```python
from build123d import *

# Parameters (mm, degrees)
SKETCH_W     = 60.2
SKETCH_H     = 8.2
PAD_DEPTH    = 0.7
SKETCH001_R  = 1
POCKET_DEPTH = 0.701
SKETCH002_W  = 8.2
SKETCH002_H  = 8.2
PAD001_DEPTH = 3
SKETCH003_R  = 3.25
PAD002_DEPTH = 5.6
SKETCH004_R  = 5
PAD003_DEPTH = 2.4
SKETCH005_R  = 4.5
PAD004_DEPTH = 0.6
SKETCH006_W  = 6.08
SKETCH006_H  = 7.5
PAD005_DEPTH = 3.2


with BuildPart() as part:
    # Sketch → Pad (new body)
    with BuildSketch(Plane.XY):
        Rectangle(SKETCH_W, SKETCH_H)
    extrude(amount=PAD_DEPTH)

    # Sketch001 → Pocket (cut, through all)
    with BuildSketch(Plane.XY.offset(0.7)):
        with Locations((-28.1, 2.1)):
            Circle(SKETCH001_R)
        with Locations((-28.1, -2.1)):
            Circle(SKETCH001_R)
        with Locations((22.4, 2.1)):
            Circle(SKETCH001_R)
    extrude(amount=-POCKET_DEPTH, mode=Mode.SUBTRACT)

    # Sketch002 → Pad001 (new body)
    with BuildSketch(Plane.XY.offset(0.7)):
        with Locations((2.4, 0)):
            Rectangle(SKETCH002_W, SKETCH002_H)
    extrude(amount=PAD001_DEPTH)

    # Sketch003 → Pad002 (new body)
    with BuildSketch(Plane.XY.offset(3.7)):
        with Locations((2.4, 0)):
            Circle(SKETCH003_R)
    extrude(amount=PAD002_DEPTH)

    # Sketch004 → Pad003 (new body)
    with BuildSketch(Plane.XY.offset(9.3)):
        with Locations((2.4, 0)):
            Circle(SKETCH004_R)
    extrude(amount=PAD003_DEPTH)

    # Sketch005 → Pad004 (new body)
    with BuildSketch(Plane.XY.offset(11.7)):
        with Locations((2.4, 0)):
            Circle(SKETCH005_R)
    extrude(amount=PAD004_DEPTH)

    # Sketch006 → Pad005 (new body)
    with BuildSketch(Plane.XY.offset(0.7)):
        with Locations((29.64, 0)):
            Rectangle(SKETCH006_W, SKETCH006_H)
    extrude(amount=PAD005_DEPTH)


solid = part.part
```
Can you work these out from the model? Positions are in its coordinate system, mm. A direction names the side the tool comes from. Coordinates: 2 decimals unless noted, no trailing zeros. Loops run counter-clockwise (first coordinate to the right, second up) from the corner with the lowest first, then second, coordinate; pieces in that order, holes last.
1) Imagine slicing it at B-B on z = 1.25. List the corners of the cut face in (x, y) for me.
2) For pin 1 (2.5 mm diameter, centred on x = 21, y = -0.5, fed in from +Z); pin 2 (1.8 mm diameter, centred on x = -11.5, z = 2.5, fed in from -Y); pin 3 (3 mm diameter, centred on x = -4, z = 1, fed in from +Y); pin 4 (2.5 mm diameter, centred on y = 1.5, z = 2.5, fed in from -X), each with a flat end and sliding along its axis, tell me the tip position at first contact or that it passes through.
3) Imagine slicing it at C-C on y = -2.1. List the corners of the cut face in (x, z) for me, plus the area to 3 significant figures.
4) Which directions (+Z, -Z, +X, -X, +Y, -Y) give clear straight access to the entire face, cutting with the end or side of a thin tool? Please do faces 1 (the flat face through (6.5, 0, 2)), 2 (the flat face through (30, 3.75, 2)), 3 (the flat face through (4, 3, 3.7)).
5) Thinking about a two-plate mould opening in Z: for faces 4 (the cylindrical face through (-27.146, 2.4, 0.355)), 5 (the cylindrical face through (5.5, 0.98, 6.46)), 6 (the flat face through (2, 0, 12.3)), which applies, pulls with the +Z half, pulls with the -Z half, needs draft (parallel to the pull), parting line crosses it, or undercut?
6) Imagine slicing it at D-D on x = 2.4. List the corners of the cut face in (y, z) for me, plus the area to 3 significant figures.
7) Imagine slicing it at A-A on x = 22.4. List the corners of the cut face in (y, z) for me, plus the area to 3 significant figures.
8) I need wall thicknesses on probe 1 along Y at (x, z) = (-28.1, 0.55); probe 2 along Y at (x, z) = (22.4, 0.5); probe 3 along Z at (x, y) = (-28, 3.75). Which ranges of each line are inside material? Lowest first, please.
Completed:
1. outline: (-1.7, -4.1) - (6.5, -4.1) - (6.5, 4.1) - (-1.7, 4.1) - close; (26.6, -3.75) - (32.68, -3.75) - (32.68, 3.75) - (26.6, 3.75) - close
2. pin 1: stops at z = 0.7
2. pin 2: passes through
2. pin 3: stops at y = 4.1
2. pin 4: stops at x = -1.7
3. outline: (-30.1, 0) - (-29.1, 0) - (-29.1, 0.7) - (-30.1, 0.7) - close; (-27.1, 0) - (30.1, 0) - (30.1, 0.7) - (32.68, 0.7) - (32.68, 3.9) - (26.6, 3.9) - (26.6, 0.7) - (6.5, 0.7) - (6.5, 3.7) - (4.88, 3.7) - (4.88, 9.3) - (6.94, 9.3) - (6.94, 11.7) - (6.38, 11.7) - (6.38, 12.3) - (-1.58, 12.3) - (-1.58, 11.7) - (-2.14, 11.7) - (-2.14, 9.3) - (-0.08, 9.3) - (-0.08, 3.7) - (-1.7, 3.7) - (-1.7, 0.7) - (-27.1, 0.7) - close
3. area: 139 mm2
4. face 1: +Y, -Y
4. face 2: +Z, +X, +Y
4. face 3: none
5. face 4: needs draft
5. face 5: undercut
5. face 6: pulls with the +Z half
6. outline: (-5, 9.3) - (-3.25, 9.3) - (-3.25, 3.7) - (-4.1, 3.7) - (-4.1, 0) - (4.1, 0) - (4.1, 3.7) - (3.25, 3.7) - (3.25, 9.3) - (5, 9.3) - (5, 11.7) - (4.5, 11.7) - (4.5, 12.3) - (-4.5, 12.3) - (-4.5, 11.7) - (-5, 11.7) - close
6. area: 96.1 mm2
7. outline: (-4.1, 0) - (1.1, 0) - (1.1, 0.7) - (-4.1, 0.7) - close; (3.1, 0) - (4.1, 0) - (4.1, 0.7) - (3.1, 0.7) - close
7. area: 4.34 mm2
8. probe 1: y = -4.1 to -3.1, -1.1 to 1.1, 3.1 to 4.1
8. probe 2: y = -4.1 to 1.1, 3.1 to 4.1
8. probe 3: z = 0 to 0.7
